Can you work these out from the model? Positions are in its coordinate system, mm. Face numbers are marked on the shaded views. A direction names the side the tool comes from. Coordinates: 2 decimals unless noted, no trailing zeros. Order: outer loops, then holes, each group sorted by start corner. A loop starts at its lowest first (then second) coordinate and runs counter-clockwise, first axis right, second up. Notation, with made-up numbers: (23.5, 74) -> (57.5, 74) arc R29 ccw to (57.5, 94) -> close; hole circle Ø5 at (27, -3.5). An arc over 180 degrees is marked (long way). Answer as a JSON object with one key per item and string values. Group by question number.
(1) Which directions (+Z, -Z, +X, -X, +Y, -Y) give clear straight access to the entire face, cutting with the end or side of a thin tool? Please do the marked faces 1 and 2.
(2) I want a section at A-A, the plane y = -30.5. List the corners of the cut face in (x, z) for me.
(3) I need wall thicknesses on line 1 (X direction, y = -27.5, z = 1); line 2 (Z direction, x = -20.5, y = -38.25); line 3 (Y direction, x = 3.5, z = 1). Which ranges of each line are inside material? Lowest first, please.
(4) For pin 1 (2 mm diameter, centred on x = 0, y = -15, fed in from +Z); pin 2 (1.6 mm diameter, centred on x = -20.5, z = 2.5, fed in from -Y), each with a flat end and sliding along its axis, tell me the tip position at first contact or that it passes through.
(5) I want a section at B-B, the plane x = -4.5. List the corners of the cut face in (y, z) for me, plus the area to 3 significant figures.
(6) If we mould it in two halves opening along X, with no side actions, what happens to the marked faces 3, 4 and 5? For each: pulls with the +X half, pulls with the -X half, needs draft (parallel to the pull), parting line crosses it, or undercut.
from build123d import *

# Parameters (mm, degrees)
F0_W     = 59
F0_H     = 79
F0_W_2   = 55
F0_H_2   = 75
F1_DEPTH = 9
F3_DEPTH = 2
F4_R     = 1
F5_DEPTH = 2.001
F6_R     = 1
F9_DEPTH = 11
F10_R    = 0.99999


# Not quite as in the source:
# - two fillets or chamfers of one size are made in one step
# - a fillet or chamfer is up to 0.001 mm smaller than in the source, because OpenCascade refuses the exact size


with BuildPart() as f1:
    # F0 (on Top) → F1 (new body)
    with BuildSketch(Plane.XY):
        Rectangle(F0_W, F0_H)
        Rectangle(F0_W_2, F0_H_2, mode=Mode.SUBTRACT)
    extrude(amount=F1_DEPTH)

    # F2 (on Top) → F3 (join)
    with BuildSketch(Plane.XY):
        Polygon((2.5, 38.5), (-2.5, 38.5), (-2.5, 2.5), (-28.5, 2.5), (-28.5, -2.5), (-2.5, -2.5), (-2.5, -38.5), (2.5, -38.5), (2.5, -2.5), (28.5, -2.5), (28.5, 2.5), (2.5, 2.5), align=None)
    extrude(amount=F3_DEPTH)

    # F4 (on face) → F5 (cut, through all)
    with BuildSketch(Plane(origin=(0, -37.5, 0), x_dir=(-1, 0, 0), z_dir=(0, 1, 0))):
        with Locations((20.5, 2.5)):
            Circle(F4_R)
        with Locations((20.5, 6.5)):
            Circle(F4_R)
        with Locations((15.5, 2.5)):
            Circle(F4_R)
        with Locations((15.5, 6.5)):
            Circle(F4_R)
    extrude(amount=-F5_DEPTH, mode=Mode.SUBTRACT)

    # F6
    f6_edges = [f1.edges().sort_by_distance(p)[0] for p in [
        (-29.5, -39.5, 4.5),
        (29.5, -39.5, 4.5),
        (-29.5, 39.5, 4.5),
        (29.5, 39.5, 4.5),
        (-2.5, 2.5, 1),
        (2.5, 2.5, 1),
        (2.5, -2.5, 1),
        (-2.5, -2.5, 1),
        (2.5, -37.5, 1),
        (-2.5, -37.5, 1),
        (-27.5, -2.5, 1),
        (-27.5, 2.5, 1),
        (27.5, -2.5, 1),
        (27.5, 2.5, 1),
        (2.5, 37.5, 1),
        (-2.5, 37.5, 1),
    ]]
    fillet(f6_edges, radius=F6_R)

    # F8 (on offset) → F9 (join)
    with BuildSketch(Plane.YZ.offset(-23.5)):
        with BuildLine():
            ThreePointArc((-37.5, 3.5), (-36.5, 4.5), (-37.5, 5.5))
            Line((-37.5, 5.5), (-37.5, 3.5))
        make_face()
    extrude(amount=F9_DEPTH)

    # F10 (radius 1 in the source; OpenCascade refuses exactly that, so slightly less here)
    f10_edges = [f1.edges().sort_by_distance(p)[0] for p in [
        (-23.5, -36.5, 4.5),
        (-12.5, -36.5, 4.5),
    ]]
    fillet(f10_edges, radius=F10_R)


solid = f1.part
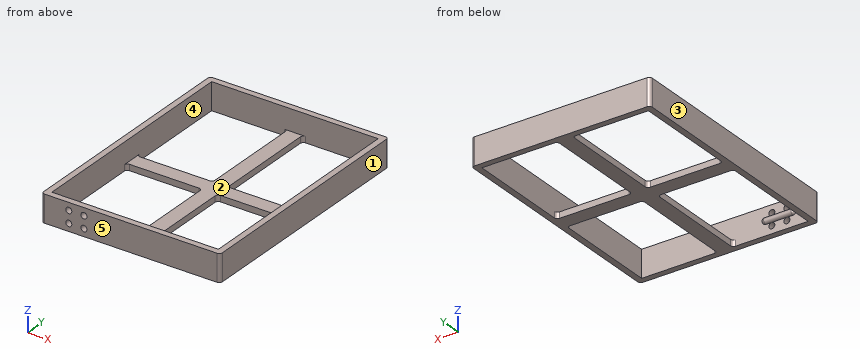
Computed values:
{
 "1": {"face 1": "+Z, -Z, +X, +Y, -Y", "face 2": "+Z"},
 "2": {"outline": "(-29.5, 0) -> (-27.5, 0) -> (-27.5, 9) -> (-29.5, 9) -> close; (-2.5, 0) -> (2.5, 0) -> (2.5, 2) -> (-2.5, 2) -> close; (27.5, 0) -> (29.5, 0) -> (29.5, 9) -> (27.5, 9) -> close"},
 "3": {"line 1": "x = -29.5 to -27.5, -2.5 to 2.5, 27.5 to 29.5", "line 2": "z = 0 to 1.5, 3.5 to 5.5, 7.5 to 9", "line 3": "y = -39.5 to -37.5, -2.5 to 2.5, 37.5 to 39.5"},
 "4": {"pin 1": "stops at z = 2", "pin 2": "stops at y = -2.5"},
 "5": {"outline": "(-39.5, 0) -> (-37.5, 0) -> (-37.5, 9) -> (-39.5, 9) -> close; (-2.5, 0) -> (2.5, 0) -> (2.5, 2) -> (-2.5, 2) -> close; (37.5, 0) -> (39.5, 0) -> (39.5, 9) -> (37.5, 9) -> close", "area": "46.0 mm2"},
 "6": {"face 3": "pulls with the -X half", "face 4": "undercut", "face 5": "needs draft"}
}
